from build123d import *

# Parameters (mm, degrees)
F1_DEPTH = 25.4
F2_R     = 12.365241
F3_DEPTH = 20.32
F5_DEPTH = 2.54


with BuildPart() as f1:
    # F0 (on Front) → F1 (new body)
    with BuildSketch(Plane.XZ):
        Polygon((22.213069, 6.299807), (35.893104, 21.369218), (25.788605, 39.036409), (5.863647, 34.885922), (3.653844, 14.653589), align=None)
    extrude(amount=F1_DEPTH)

    # F2 (on face) → F3 (cut)
    with BuildSketch(Plane.XZ.offset(25.4)):
        with Locations((19.056195, 23.6161)):
            Circle(F2_R)
    extrude(amount=-F3_DEPTH, mode=Mode.SUBTRACT)

    # F4 (on face) → F5 (join)
    with BuildSketch(Plane(origin=(2.029152, 0, -0.221627), x_dir=(0, -1, 0), z_dir=(-0.994088, 0, 0.108576))):
        Polygon((25.4, 14.963679), (25.4, 35.316332), (0, 25.140005), align=None)
    extrude(amount=F5_DEPTH)


solid = f1.part
Geometry check sheet. Reference: the model listing, model coordinates, mm. A direction names the side the tool comes from. Coordinates: 2 decimals unless noted, no trailing zeros. Order: outer loops, then holes, each group sorted by start corner. A loop starts at its lowest first (then second) coordinate and runs counter-clockwise, first axis right, second up. Notation, with made-up numbers: (40.5, 75.5) -> (79.5, 75.5) arc R8 ccw to (79.5, 81.5) -> close; hole circle Ø2 at (-5, 27.25). An arc over 180 degrees is marked (long way). Use a Markdown table: item, result. Add a question column.
1. Cross-section at D-D (y = -3.75). Enter the section's corners in (x, z), and give its area (3 significant figures).
2. Cross-section at A-A (y = -9.75). Enter the section's corners in (x, z).
3. Go/stop test with flat-tipped pins: pin 1 Ø5 at (y, z) = (-5, 32.5) entering from +X; pin 2 Ø12 at (y, z) = (-22, 35.5) entering from +X; pin 3 Ø1 at (x, y) = (13.5, -14.5) entering from -Z. Record where each tip stops, or that it passes through.
4. Set-up check for faces 4 (the face through (6.703, -15.382, 24.16)), 5 (the face through (2.97, -12.52, 19.92)), 6 (the face through (4.074, -12.878, 30.035)): record each of +Z, -Z, +X, -X, +Y, -Y from which the full face is reachable in a straight line by a thin tool's end or side.
5. Cross-section at B-B (x = 16). Enter the section's corners in (y, z).
6. Cross-section at C-C (z = 29.5). Enter the section's corners in (x, y), and give its area (3 significant figures).
7. Mould release check, pull along Z, two halves, no side actions. Record for faces 1 (the face through (19, -5.08, 24)), 2 (the face through (15.97, -12.52, 36.99)), 3 (the face through (20, 0, 23)): pulls with the +Z half, pulls with the -Z half, needs draft (parallel to the pull), parting line crosses it, or undercut.
8. Material ranges on L1, parallel to Y at x = 21, z = 13.5; L2, parallel to Z at x = 23, y = -17.5; L3, parallel to Z at x = 19, y = -23.5, recorded low to high.
Filled sheet:
| question | item | result |
|---|---|---|
| 1 | outline | (2.07, 23.55) -> (4.6, 23.28) -> (3.65, 14.65) -> (22.21, 6.3) -> (35.89, 21.37) -> (25.79, 39.04) -> (5.86, 34.89) -> (4.92, 26.26) -> (2.4, 26.54) -> close |
| 1 | area | 720 mm2 |
| 2 | outline | (1.81, 21.16) -> (4.33, 20.89) -> (3.65, 14.65) -> (22.21, 6.3) -> (35.89, 21.37) -> (25.79, 39.04) -> (5.86, 34.89) -> (5.18, 28.65) -> (2.66, 28.93) -> close; hole circle Ø24.73 at (19.06, 23.62) |
| 3 | pin 1 | x = 30.96 |
| 3 | pin 2 | x = 31.24 |
| 3 | pin 3 | z = 10 |
| 4 | face 4 | -Y |
| 4 | face 5 | -X, +Y |
| 4 | face 6 | +Z, +Y |
| 5 | outline | (-25.4, 9.1) -> (0, 9.1) -> (0, 37) -> (-25.4, 37) -> (-25.4, 35.6) -> (-5.08, 35.6) -> (-5.08, 11.63) -> (-25.4, 11.63) -> close |
| 6 | outline | (2.72, -25.4) -> (8.18, -25.4) -> (8.18, -5.08) -> (29.93, -5.08) -> (29.93, -25.4) -> (31.24, -25.4) -> (31.24, 0) -> (5.28, 0) -> (5.28, -11.88) -> (2.72, -11.18) -> close |
| 6 | area | 253 mm2 |
| 7 | face 1 | undercut |
| 7 | face 2 | pulls with the +Z half |
| 7 | face 3 | needs draft |
| 8 | L1 | -5.08 to 0 |
| 8 | L2 | 7.17 to 11.9, 35.34 to 38.46 |
| 8 | L3 | 7.75 to 11.25, 35.98 to 37.62 |
